Can you work these out from the model? Positions are in its coordinate system, mm. Give positions to 0.01 mm unless a question says otherwise; leave off trailing zeros. Write each loop counter-clockwise with the first axis right and the second up, starting at its lowest first coordinate (ties: lowest second). Pieces come first, ordered by that corner, then holes. Notation, with made-up numbers: (65, -3) -> (93, -3) arc R36 cw to (93, 34) -> close; hole circle Ø10 at (-34, -25). An arc over 180 degrees is marked (long way). One line per item, written item: value.
from build123d import *

# Parameters (mm, degrees)
SKETCH1_W               = 200
SKETCH1_H               = 100
BOSS_EXTRUDE1_DEPTH     = 12
CUT_EXTRUDE1_REACH      = 114.446
SKETCH2_R               = 7
FILL_PATTERN1_OUTLINE_R = 7
FILL_PATTERN1_DEPTH     = 12


# Read off the part's stored shape, not the designer's step: Fill Pattern1
with BuildPart() as part:
    # Sketch1 → Boss-Extrude1 (new body)
    with BuildSketch(Plane.XY):
        Rectangle(SKETCH1_W, SKETCH1_H)
    extrude(amount=BOSS_EXTRUDE1_DEPTH)

    # Sketch2 → Cut-Extrude1 (cut, up to next)
    with BuildSketch(Plane.XY.offset(12), mode=Mode.PRIVATE) as cut_extrude1_sk1:
        Circle(SKETCH2_R)
    cut_extrude1_tool1 = extrude(cut_extrude1_sk1.sketch, amount=-CUT_EXTRUDE1_REACH, mode=Mode.PRIVATE) & part.part
    add(cut_extrude1_tool1.solids().sort_by_distance((0, 0, 12))[0], mode=Mode.SUBTRACT)

    # Fill Pattern1 outline → Fill Pattern1 (cut)
    with BuildSketch(Plane.XY):
        with Locations((-39.656562733, 33.666424355)):
            Circle(FILL_PATTERN1_OUTLINE_R)
        with Locations((39.656562733, -33.666424355)):
            Circle(FILL_PATTERN1_OUTLINE_R)
        with Locations((59.484844099, -25.249818266)):
            Circle(FILL_PATTERN1_OUTLINE_R)
        with Locations((79.313125466, -16.833212178)):
            Circle(FILL_PATTERN1_OUTLINE_R)
        with Locations((19.828281366, 25.249818266)):
            Circle(FILL_PATTERN1_OUTLINE_R)
        with Locations((0, 16.833212178)):
            Circle(FILL_PATTERN1_OUTLINE_R)
        with Locations((-19.828281366, 8.416606089)):
            Circle(FILL_PATTERN1_OUTLINE_R)
        with Locations((-39.656562733, 0)):
            Circle(FILL_PATTERN1_OUTLINE_R)
        with Locations((-59.484844099, -8.416606089)):
            Circle(FILL_PATTERN1_OUTLINE_R)
        with Locations((-79.313125466, -16.833212178)):
            Circle(FILL_PATTERN1_OUTLINE_R)
        with Locations((59.484844099, 25.249818266)):
            Circle(FILL_PATTERN1_OUTLINE_R)
        with Locations((39.656562733, 16.833212178)):
            Circle(FILL_PATTERN1_OUTLINE_R)
        with Locations((-59.484844099, 25.249818266)):
            Circle(FILL_PATTERN1_OUTLINE_R)
        with Locations((-79.313125466, 16.833212178)):
            Circle(FILL_PATTERN1_OUTLINE_R)
        with Locations((0, 33.666424355)):
            Circle(FILL_PATTERN1_OUTLINE_R)
        with Locations((-19.828281366, 25.249818266)):
            Circle(FILL_PATTERN1_OUTLINE_R)
        with Locations((39.656562733, 33.666424355)):
            Circle(FILL_PATTERN1_OUTLINE_R)
        with Locations((-79.313125466, 0)):
            Circle(FILL_PATTERN1_OUTLINE_R)
        with Locations((-59.484844099, 8.416606089)):
            Circle(FILL_PATTERN1_OUTLINE_R)
        with Locations((-39.656562733, 16.833212178)):
            Circle(FILL_PATTERN1_OUTLINE_R)
        with Locations((79.313125466, 0)):
            Circle(FILL_PATTERN1_OUTLINE_R)
        with Locations((-39.656562733, -33.666424355)):
            Circle(FILL_PATTERN1_OUTLINE_R)
        with Locations((-19.828281366, -25.249818266)):
            Circle(FILL_PATTERN1_OUTLINE_R)
        with Locations((0, -16.833212178)):
            Circle(FILL_PATTERN1_OUTLINE_R)
        with Locations((59.484844099, -8.416606089)):
            Circle(FILL_PATTERN1_OUTLINE_R)
        with Locations((39.656562733, -16.833212178)):
            Circle(FILL_PATTERN1_OUTLINE_R)
        with Locations((19.828281366, -25.249818266)):
            Circle(FILL_PATTERN1_OUTLINE_R)
        with Locations((0, -33.666424355)):
            Circle(FILL_PATTERN1_OUTLINE_R)
        with Locations((19.828281366, 8.416606089)):
            Circle(FILL_PATTERN1_OUTLINE_R)
        with Locations((-19.828281366, -8.416606089)):
            Circle(FILL_PATTERN1_OUTLINE_R)
        with Locations((-39.656562733, -16.833212178)):
            Circle(FILL_PATTERN1_OUTLINE_R)
        with Locations((-59.484844099, -25.249818266)):
            Circle(FILL_PATTERN1_OUTLINE_R)
        with Locations((79.313125466, 16.833212178)):
            Circle(FILL_PATTERN1_OUTLINE_R)
        with Locations((59.484844099, 8.416606089)):
            Circle(FILL_PATTERN1_OUTLINE_R)
        with Locations((39.656562733, 0)):
            Circle(FILL_PATTERN1_OUTLINE_R)
        with Locations((19.828281366, -8.416606089)):
            Circle(FILL_PATTERN1_OUTLINE_R)
    extrude(amount=FILL_PATTERN1_DEPTH, mode=Mode.SUBTRACT)


solid = part.part
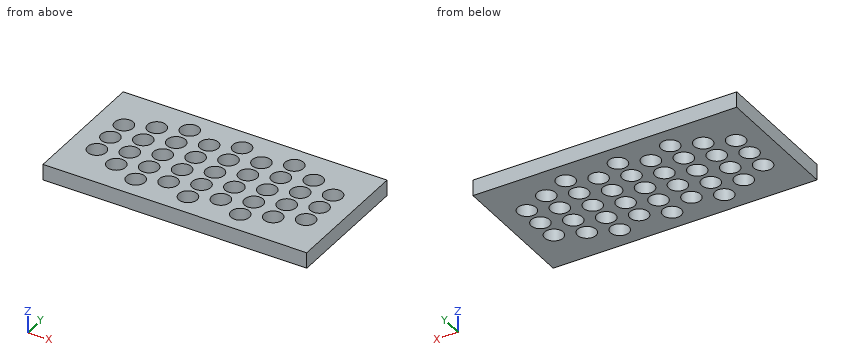
1) If we section it at C-C (y = -29): State how many separate pieces and enclosed holes the cut face has, and give its area (3 significant figures).
Answer list:
separate pieces: 8
enclosed holes: 0
area: 1,460 mm^2
2) If we section it at B-B (x = -74.5): Write out the boundary of the cut face in (y, z), and give its area (3 significant figures).
Answer list:
outline: (-50, 0) -> (-21.92, 0) -> (-21.92, 12) -> (-50, 12) -> close; (-11.75, 0) -> (-5.08, 0) -> (-5.08, 12) -> (-11.75, 12) -> close; (5.08, 0) -> (11.75, 0) -> (11.75, 12) -> (5.08, 12) -> close; (21.92, 0) -> (50, 0) -> (50, 12) -> (21.92, 12) -> close
area: 834 mm^2
3) If we section it at A-A (x = 0): Write out the boundary of the cut face in (y, z).
Answer list:
outline: (-50, 0) -> (-40.67, 0) -> (-40.67, 12) -> (-50, 12) -> close; (-26.67, 0) -> (-23.83, 0) -> (-23.83, 12) -> (-26.67, 12) -> close; (-9.83, 0) -> (-7, 0) -> (-7, 12) -> (-9.83, 12) -> close; (7, 0) -> (9.83, 0) -> (9.83, 12) -> (7, 12) -> close; (23.83, 0) -> (26.67, 0) -> (26.67, 12) -> (23.83, 12) -> close; (40.67, 0) -> (50, 0) -> (50, 12) -> (40.67, 12) -> close
4) If we section it at D-D (x = 77): Write out the boundary of the cut face in (y, z).
Answer list:
outline: (-50, 0) -> (-23.44, 0) -> (-23.44, 12) -> (-50, 12) -> close; (-10.23, 0) -> (-6.61, 0) -> (-6.61, 12) -> (-10.23, 12) -> close; (6.61, 0) -> (10.23, 0) -> (10.23, 12) -> (6.61, 12) -> close; (23.44, 0) -> (50, 0) -> (50, 12) -> (23.44, 12) -> close
5) I need wall thicknesses on L1, parallel to X at y = 33.5, z = 4.25; L2, parallel to Y at x = 60, z = 8.5; L3, parallel to X at y = -17, z = 10.25. Which ranges of each line are inside material? Lowest first, please.
Answer list:
L1: x = -100 to -46.65, -32.66 to -7, 7 to 32.66, 46.65 to 100
L2: y = -50 to -32.23, -18.27 to -15.4, -1.44 to 1.44, 15.4 to 18.27, 32.23 to 50
L3: x = -100 to -86.31, -72.32 to -46.65, -32.66 to -7, 7 to 32.66, 46.65 to 72.32, 86.31 to 100
